from build123d import *

# Parameters (mm, degrees)
SKETCH015_W             = 42
SKETCH015_H             = 32
PAD003_DEPTH            = 1.6
SKETCH016_W             = 35.8
SKETCH016_H             = 32
PAD004_DEPTH            = 1.75
SKETCH017_R             = 1.25
PAD005_DEPTH            = 1.6
SKETCH018_W             = 13
SKETCH018_H             = 5
SKETCH018_W_2           = 15
SKETCH018_H_2           = 12
PAD006_DEPTH            = 1.7
BODY002_PLACEMENT_ANGLE = 90


with BuildPart() as part:
    # Sketch015 → Pad003 (new body)
    with BuildSketch(Plane.XY):
        Rectangle(SKETCH015_W, SKETCH015_H)
    extrude(amount=PAD003_DEPTH)

    # Sketch016 (on Face6 of Pad003) → Pad004 (join)
    with BuildSketch(Plane.XY.offset(1.6)):
        with Locations((2.5, 0)):
            Rectangle(SKETCH016_W, SKETCH016_H)
    extrude(amount=PAD004_DEPTH)

    # Sketch017 (on Face3 of Pad004) → Pad005 (join)
    with BuildSketch(Plane.XY.offset(1.6)):
        with BuildLine():
            Line((-21, 16), (-15.95, 16))
            Line((-15.95, 16), (-15.95, 18.575))
            ThreePointArc((-15.95, 18.575), (-16.689555, 20.360445), (-18.475, 21.1))
            ThreePointArc((-18.475, 21.1), (-20.260445, 20.360445), (-21, 18.575))
            Line((-21, 18.575), (-21, 16))
        make_face()
        with Locations((-18.475, 18.575)):
            Circle(SKETCH017_R, mode=Mode.SUBTRACT)
        with BuildLine():
            Line((15.95, 16), (21, 16))
            Line((21, 16), (21, 18.575))
            ThreePointArc((21, 18.575), (20.260445, 20.360445), (18.475, 21.1))
            ThreePointArc((18.475, 21.1), (16.689555, 20.360445), (15.95, 18.575))
            Line((15.95, 18.575), (15.95, 16))
        make_face()
        with Locations((18.475, 18.575)):
            Circle(SKETCH017_R, mode=Mode.SUBTRACT)
        with BuildLine():
            Line((-21, -16), (-15.95, -16))
            Line((-15.95, -16), (-15.95, -18.575))
            ThreePointArc((-18.475, -21.1), (-16.689555, -20.360445), (-15.95, -18.575))
            ThreePointArc((-21, -18.575), (-20.260445, -20.360445), (-18.475, -21.1))
            Line((-21, -18.575), (-21, -16))
        make_face()
        with Locations((-18.475, -18.575)):
            Circle(SKETCH017_R, mode=Mode.SUBTRACT)
        with BuildLine():
            Line((15.95, -16), (21, -16))
            Line((21, -16), (21, -18.575))
            ThreePointArc((18.475, -21.1), (20.260445, -20.360445), (21, -18.575))
            ThreePointArc((15.95, -18.575), (16.689555, -20.360445), (18.475, -21.1))
            Line((15.95, -18.575), (15.95, -16))
        make_face()
        with Locations((18.475, -18.575)):
            Circle(SKETCH017_R, mode=Mode.SUBTRACT)
    extrude(amount=-PAD005_DEPTH)

    # Sketch018 (on Face15 of Pad005) → Pad006 (join)
    with BuildSketch(Plane(origin=(0, 0, 0), x_dir=(1, 0, 0), z_dir=(0, 0, -1))):
        with Locations((-6.5, -12.5)):
            Rectangle(SKETCH018_W, SKETCH018_H)
        with Locations((11.5, -8)):
            Rectangle(SKETCH018_W_2, SKETCH018_H_2)
    extrude(amount=PAD006_DEPTH)


with BuildPart() as part_1:
    # Body002 placement: moved
    add(part.part.moved(Location((0, 13, 21.75))).rotate(Axis((0, 13, 21.75), (0, 0, -1)), BODY002_PLACEMENT_ANGLE))


solid = part_1.part
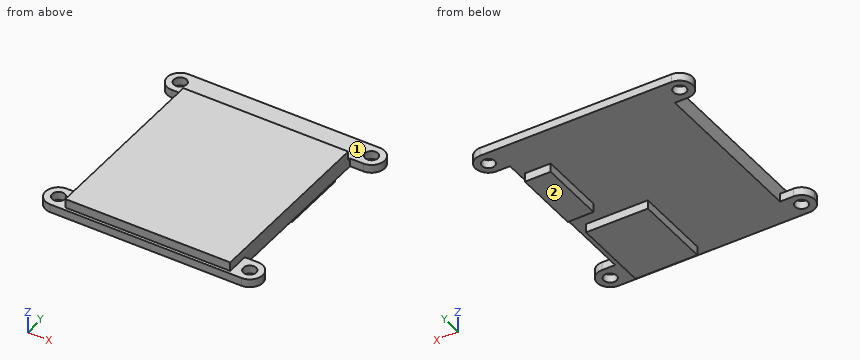
Read the model definition and answer for the solid it produces. Units are mm, in the model's axes. Face numbers are marked on the shaded views. A direction names the side the tool comes from. Give positions to 0.01 mm unless a question says otherwise; leave off trailing zeros. Write each loop counter-clockwise with the first axis right and the second up, starting at its lowest first coordinate (ties: lowest second). Pieces come first, ordered by that corner, then holes. Notation, with made-up numbers: (-17, -22.5) - (24, -22.5) arc R10 ccw to (24, -13.5) - close; hole circle Ø7 at (7, 12). An arc over 180 degrees is marked (long way). Answer in a Markdown table with one row per item. Add a question column.
Item 1: Section B-B, the plane x = 1.5 is taken. Write down the section's boundary in (y, z).
Item 2: Section D-D, the plane z = 24.6 is taken. Write down the section's boundary in (x, y).
Item 3: Find the intervals of material crossed by L1, parallel to X at y = 32.5, z = 22.05; L2, parallel to Y at x = -17.5, z = 23; L3, parallel to Y at x = 16.5, z = 23.25, in increasing order.
Item 4: Section C-C, the plane y = 19 is taken. Write down the section's boundary in (x, z), and give its area (3 significant figures).
Item 5: Section A-A, the plane z = 20.6 is taken. Write down the section's boundary in (x, y), and give its area (3 significant figures).
Item 6: A tool of negligible diameter and unlimited length cuts with its end or side. For the marked faces 1 and 2, from which of +Z, -Z, +X, -X, +Y, -Y can it reach the whole face along a straight path? Write none if from no direction.
Item 7: Flat-ended cylindrical pins translate along their axes: P1, Ø2.5, axis at y = 14, z = 24, coming from the +X side; P2, Ø1, axis at y = 4.5, z = 23, coming from the -X side; P3, Ø4, axis at x = 18.575, y = 31.475, coming from the +Z side; P4, Ø1.9, axis at x = -5, z = 24, coming from the +Y side. Find the tip coordinate at first contact, or state that the pin passes through.
Recorded:
| question | item | result |
|---|---|---|
| 1 | outline | (-8, 21.75) - (34, 21.75) - (34, 23.35) - (28.4, 23.35) - (28.4, 25.1) - (-7.4, 25.1) - (-7.4, 23.35) - (-8, 23.35) - close |
| 2 | outline | (-16, -7.4) - (16, -7.4) - (16, 28.4) - (-16, 28.4) - close |
| 3 | L1 | x = -20.88 to -19.29, -17.86 to 17.86, 19.29 to 20.88 |
| 3 | L2 | y = -8 to -6.11, -4.84 to -2.95, 28.95 to 30.84, 32.11 to 34 |
| 3 | L3 | y = -8 to -2.95, 28.95 to 34 |
| 4 | outline | (-16, 21.75) - (10, 21.75) - (10, 20.05) - (15, 20.05) - (15, 21.75) - (16, 21.75) - (16, 25.1) - (-16, 25.1) - close |
| 4 | area | 116 mm2 |
| 5 | outline | (2, -6) - (14, -6) - (14, 9) - (2, 9) - close; (10, 13) - (15, 13) - (15, 26) - (10, 26) - close |
| 5 | area | 245 mm2 |
| 6 | face 1 | +Z, +X, -X, +Y |
| 6 | face 2 | -Z, +X, -X, +Y, -Y |
| 7 | P1 | stops at x = 16 |
| 7 | P2 | stops at x = -16 |
| 7 | P3 | stops at z = 23.35 |
| 7 | P4 | stops at y = 34 |
